Read the model definition and answer for the solid it produces. Units are mm, in the model's axes. Coordinates: 2 decimals unless noted, no trailing zeros. Loops run counter-clockwise (first coordinate to the right, second up) from the corner with the lowest first, then second, coordinate; pieces in that order, holes last. Notation, with made-up numbers: (-26, -38) -> (0, -38) arc R18 ccw to (0, -18) -> close; hole circle Ø2 at (25.5, 25). An arc over 180 degrees is marked (long way). Answer in a Markdown table with one row per item.
```python
from build123d import *

# Parameters (mm, degrees)
BOSS_EXTRUDE1_DEPTH = 3.175
FILLET1_R           = 12.7
FILLET2_R           = 1.5875
FILLET3_R           = 1.5875
SKETCH2_R           = 2.032
CUT_EXTRUDE1_DEPTH  = 69.535995798
FILLET4_R           = 1.5875


with BuildPart() as part:
    # Sketch1 → Boss-Extrude1 (new body)
    with BuildSketch(Plane(origin=(0, 0, 0), x_dir=(0, 0, -1), z_dir=(1, 0, 0))):
        with BuildLine():
            Line((13.748153285, 22.0345), (14.739116884, 20.318100699))
            ThreePointArc((14.739116884, 20.318100699), (14.158051555, 18.149535371), (16.326616884, 17.568470042))
            ThreePointArc((16.326616884, 17.568470042), (19.207719521, 21.158249529), (18.906671331, 25.751357318))
            Line((18.906671331, 25.751357318), (17.516713222, 28.732132102))
            ThreePointArc((17.516713222, 28.732132102), (10.661882173, 37.091365139), (0.634495892, 41.130797035))
            Line((0.634495892, 41.130797035), (-40.382266976, 46.59538876))
            Line((-40.382266976, 46.59538876), (-50.475527532, 44.45))
            Line((-50.475527532, 44.45), (-31.992178218, -42.507321705))
            Line((-31.992178218, -42.507321705), (-21.898917663, -40.361932946))
            Line((-21.898917663, -40.361932946), (-27.991294866, -5.810344877))
            Line((-27.991294866, -5.810344877), (-10.998522628, 23.622))
            ThreePointArc((-10.998522628, 23.622), (-6.35, 28.270522628), (0, 29.972))
            ThreePointArc((0, 29.972), (7.9375, 27.845153285), (13.748153285, 22.0345))
        make_face()
    extrude(amount=BOSS_EXTRUDE1_DEPTH)

    # Fillet1
    fillet1_edges = [part.edges().sort_by_distance(p)[0] for p in [
        (1.5875, -5.810344877, 27.991294866),
    ]]
    fillet(fillet1_edges, radius=FILLET1_R)

    # Fillet2
    fillet2_edges = [part.edges().sort_by_distance(p)[0] for p in [
        (1.5875, -40.361932946, 21.898917663),
        (1.5875, -42.507321705, 31.992178218),
        (1.5875, 44.45, 50.475527532),
        (1.5875, 46.59538876, 40.382266976),
    ]]
    fillet(fillet2_edges, radius=FILLET2_R)

    # Fillet3
    fillet3_edges = [part.edges().sort_by_distance(p)[0] for p in [
        (1.5875, 20.318100699, -14.739116884),
    ]]
    fillet(fillet3_edges, radius=FILLET3_R)

    # Sketch2 → Cut-Extrude1 (cut, through all)
    with BuildSketch(Plane(origin=(3.175, 0, 0), x_dir=(0, 0, -1), z_dir=(1, 0, 0))):
        with Locations((-43.17662111, 33.017704898)):
            Circle(SKETCH2_R)
        with Locations((-29.974228743, -29.094667748)):
            Circle(SKETCH2_R)
        with BuildLine():
            Line((-21.848305026, 20.704625636), (-17.872599271, 27.59075))
            ThreePointArc((-17.872599271, 27.59075), (-14.903788227, 31.547275925), (-11.078768079, 34.683700207))
            Line((-11.078768079, 34.683700207), (-40.047392283, 38.543139447))
            ThreePointArc((-40.047392283, 38.543139447), (-37.495523437, 35.854539267), (-36.879589172, 32.199237568))
            Line((-36.879589172, 32.199237568), (-21.848305026, 20.704625636))
        make_face()
        with BuildLine():
            Line((-38.286199293, 25.280985715), (-25.05001183, 15.159106781))
            Line((-25.05001183, 15.159106781), (-32.554160521, 2.161539981))
            ThreePointArc((-32.554160521, 2.161539981), (-32.855452365, 1.621137898), (-33.140409238, 1.071946887))
            Line((-33.140409238, 1.071946887), (-38.286199293, 25.280985715))
        make_face()
    extrude(amount=-CUT_EXTRUDE1_DEPTH, mode=Mode.SUBTRACT)

    # Fillet4
    fillet4_edges = [part.edges().sort_by_distance(p)[0] for p in [
        (1.5875, 20.704625636, 21.848305026),
        (1.5875, 34.683700207, 11.078768079),
        (1.5875, 38.543139447, 40.047392283),
        (1.5875, 32.199237568, 36.879589172),
        (1.5875, 25.280985715, 38.286199293),
        (1.5875, 1.071946887, 33.140409238),
        (1.5875, 15.159106781, 25.05001183),
    ]]
    fillet(fillet4_edges, radius=FILLET4_R - 0.0001)  # a hair under: the kernel refuses the full size


solid = part.part
```
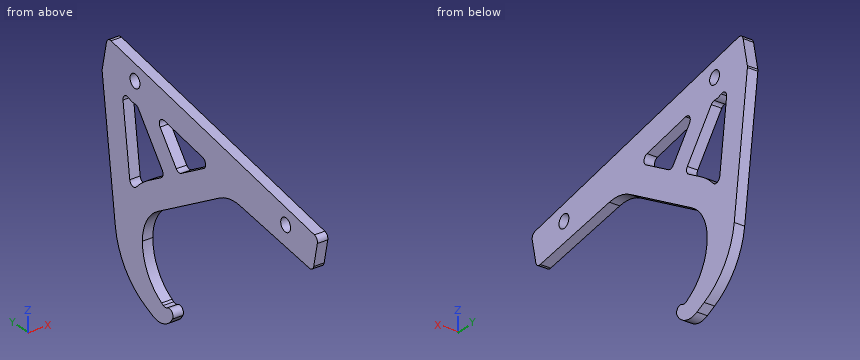
1. Given pin 1 Ø2.5 at (y, z) = (-29.09, 29.97) entering from +X; pin 2 Ø6 at (y, z) = (32, 37.5) entering from -X; pin 3 Ø1 at (x, y) = (1.5, -27) entering from -Z, each flat-ended and moving along its own axis, determine where each tip first touches the part or whether it passes through.
A:
| item | result |
|---|---|
| pin 1 | passes through |
| pin 2 | stops at x = 0 |
| pin 3 | stops at z = 24.17 |
2. A cutting plane is placed at B-B on y = -28. Give the vertices of the cut face in (x, z) (3 decimals), and give its area (3 significant figures).
A:
| item | result |
|---|---|
| outline | (0, 24.079) -> (3.175, 24.079) -> (3.175, 28.262) -> (0, 28.262) -> close; (0, 31.686) -> (3.175, 31.686) -> (3.175, 35.076) -> (0, 35.076) -> close |
| area | 24.0 mm2 |
3. A cutting plane is placed at A-A on z = 24.5. Give the vertices of the cut face in (x, y) (3 decimals).
A:
| item | result |
|---|---|
| outline | (0, -40.915) -> (3.175, -40.915) -> (3.175, -25.61) -> (0, -25.61) -> close; (0, 0.237) -> (3.175, 0.237) -> (3.175, 22.732) -> (0, 22.732) -> close; (0, 36.472) -> (3.175, 36.472) -> (3.175, 44.479) -> (0, 44.479) -> close |
4. A cutting plane is placed at C-C on x = 1.7. Count the separate pieces of the cut face and the enclosed holes in it, and give its area (3 significant figures).
A:
| item | result |
|---|---|
| separate pieces | 1 |
| enclosed holes | 4 |
| area | 1,870 mm2 |
5. A cutting plane is placed at D-D on z = 1.5. Give the vertices of the cut face in (x, y) (3 decimals), and give its area (3 significant figures).
A:
| item | result |
|---|---|
| outline | (0, 29.883) -> (3.175, 29.883) -> (3.175, 41.415) -> (0, 41.415) -> close |
| area | 36.6 mm2 |
6. Find the intervals of material crossed by probe 1 along Z at (x, y) = (1.45, 18) (3 decimals); probe 2 along Y at (x, z) = (2.9, 16); probe 3 along Z at (x, y) = (1.65, 8), in increasing order.
A:
| item | result |
|---|---|
| probe 1 | z = -16.978 to -14.256, 14.244 to 28.765, 36.739 to 44.853 |
| probe 2 | y = 14.96 to 30.31, 35.34 to 43.35 |
| probe 3 | z = 20.02 to 29.18, 34.61 to 42.73 |
